Source: CAD feature listing. Evaluate the final solid. Frame: model axes, mm. A direction names the side the tool comes from. Give positions to 0.01 mm unless a question says otherwise; leave off trailing zeros. Write each loop counter-clockwise with the first axis right and the second up, starting at its lowest first coordinate (ties: lowest second). Pieces come first, ordered by that corner, then holes. Notation, with made-up numbers: (70.25, 42) -> (81.25, 42) arc R16 cw to (81.25, 56) -> close; hole circle Ø6 at (55, 82). An arc over 180 degrees is marked (long way). Use a Markdown table: item, result. Add a question column.
```python
from build123d import *

# Parameters (mm, degrees)
BOSS_EXTRUDE1_DEPTH = 45
BOSS_EXTRUDE2_START = -40
SKETCH1_3_R         = 10
BOSS_EXTRUDE2_DEPTH = 86
SKETCH1_4_R         = 10
BOSS_EXTRUDE3_DEPTH = 40
SKETCH1_5_R         = 25
BOSS_EXTRUDE4_DEPTH = 20
SKETCH2_R           = 5
BOSS_EXTRUDE5_DEPTH = 60
BOSS_EXTRUDE6_DEPTH = 10
SKETCH4_R           = 8
CUT_EXTRUDE2_DEPTH  = 15


with BuildPart() as part:
    # Sketch1 → Boss-Extrude1 (new body)
    with BuildSketch(Plane.XY):
        Polygon((15.533008589, 37.5), (-15.533008589, 37.5), (-37.5, 15.533008589), (-37.5, -15.533008589), (-15.533008589, -37.5), (15.533008589, -37.5), (37.5, -15.533008589), (37.5, 15.533008589), align=None)
    extrude(amount=BOSS_EXTRUDE1_DEPTH)

    # Sketch1<3> → Boss-Extrude2 (add)
    with BuildSketch(Plane.XY.offset(BOSS_EXTRUDE2_START)):
        with Locations((-15, 0)):
            Circle(SKETCH1_3_R)
    boss_extrude2 = extrude(amount=BOSS_EXTRUDE2_DEPTH)

    # Sketch1<4> → Boss-Extrude3 (add)
    with BuildSketch(Plane.XY):
        with Locations((15, 0)):
            Circle(SKETCH1_4_R)
    extrude(amount=-BOSS_EXTRUDE3_DEPTH)

    # Sketch1<5> → Boss-Extrude4 (add)
    with BuildSketch(Plane.XY):
        Circle(SKETCH1_5_R)
    extrude(amount=-BOSS_EXTRUDE4_DEPTH)

    # Sketch2 → Boss-Extrude5 (add)
    with BuildSketch(Plane(origin=(0, 0, -40), x_dir=(-1, 0, 0), z_dir=(0, 0, -1))):
        with Locations((15, 0)):
            Circle(SKETCH2_R)
    boss_extrude5 = extrude(amount=BOSS_EXTRUDE5_DEPTH)

    # Mirror2: Boss-Extrude5 across plane
    add(boss_extrude5.mirror(Plane(origin=(0, 0, 0), x_dir=(0, 0, 1), z_dir=(1, 0, 0))))

    # Sketch3 → Boss-Extrude6 (add)
    with BuildSketch(Plane(origin=(0, 0, -100), x_dir=(-1, 0, 0), z_dir=(0, 0, -1))):
        Polygon((-6.882058498, 0), (-9.259748515, 5.740251485), (-15, 8.117941502), (-20.740251485, 5.740251485), (-23.117941502, 0), (-20.740251485, -5.740251485), (-15, -8.117941502), (-9.259748515, -5.740251485), align=None)
    boss_extrude6 = extrude(amount=BOSS_EXTRUDE6_DEPTH)

    # Mirror3: Boss-Extrude6 across plane
    add(boss_extrude6.mirror(Plane(origin=(0, 0, 0), x_dir=(0, 0, 1), z_dir=(1, 0, 0))))

    # Mirror4: Boss-Extrude2 across plane
    add(boss_extrude2.mirror(Plane(origin=(0, 0, 0), x_dir=(0, 0, 1), z_dir=(1, 0, 0))))

    # Sketch4 → Cut-Extrude2 (cut)
    with BuildSketch(Plane.XY.offset(46)):
        with Locations((-15, 0)):
            Circle(SKETCH4_R)
    cut_extrude2 = extrude(amount=-CUT_EXTRUDE2_DEPTH, mode=Mode.SUBTRACT)

    # Mirror5: Cut-Extrude2 across plane
    add(cut_extrude2.mirror(Plane(origin=(0, 0, 0), x_dir=(0, 0, 1), z_dir=(1, 0, 0))), mode=Mode.SUBTRACT)


solid = part.part
```
(1) Cut plane A-A on x = 0. Return the cut outline in (y, z), then the cut area to 4 significant figures.
(2) Cut plane B-B on z = 24. Return the cut outline in (x, y), then the cut area to 3 significant figures.
(3) First-contact query: pin 1 Ø8 at (x, z) = (-22, 16) entering from +Y; pin 2 Ø10 at (y, z) = (-3, -75) entering from -X; pin 3 Ø12 at (y, z) = (14, -53) entering from +X; pin 4 Ø6 at (y, z) = (-24, -20.5) entering from -X. Flat tips, straight axial feed; report the tip coordinate or a pass-through.
(4) Cut plane C-C on z = -74. Return the cut outline in (x, y), then the cut area to 3 significant figures.
(5) Cut plane D-D on x = -17.5. Return the cut outline in (y, z), then the cut area to 3 significant figures.
(6) Access query for faces 1 (the flat face through (8.088, -2.91, -104.93)), 2 (the flat face through (-21.912, 2.91, -104.93)), 3 (the flat face through (17.83, 6.946, -104.93)), 4 (the cylindrical face through (-19.77, 1.5, -69.58)), 5 (the flat face through (-8.054, 2.83, -104.93)). Directions: +Z, -Z, +X, -X, +Y, -Y. A direction counts if a zero-diameter tool reaches every point of the face in a straight line with its end or side. Return the directions, or none.
(7) Mould query, pull axis Z, two halves, no side actions, for faces 6 (the flat face through (15, 0, 31)), 7 (the cylindrical face through (-5.46, 3, -30.14)), 8 (the flat face through (-13, 5, -40)). Classes: +Z half, -Z half, draft (parallel to the pull), parting line (faces both ways), or undercut.
(8) Material intervals for L1, parallel to Y at x = 15, z = 38.75; L2, parallel to Z at x = 17.5, y = -6.5; L3, parallel to Z at x = 1, y = 29, sorted ascending.
Output:
| question | item | result |
|---|---|---|
| 1 | outline | (-37.5, 0) -> (-25, 0) -> (-25, -20) -> (25, -20) -> (25, 0) -> (37.5, 0) -> (37.5, 45) -> (-37.5, 45) -> close |
| 1 | area | 4,375 mm^2 |
| 2 | outline | (-37.5, -15.53) -> (-15.53, -37.5) -> (15.53, -37.5) -> (37.5, -15.53) -> (37.5, 15.53) -> (15.53, 37.5) -> (-15.53, 37.5) -> (-37.5, 15.53) -> close |
| 2 | area | 4,660 mm^2 |
| 3 | pin 1 | y = 35.03 |
| 3 | pin 2 | x = -20 |
| 3 | pin 3 | through |
| 3 | pin 4 | x = -13.5 |
| 4 | outline | circle Ø10 at (-15, 0); circle Ø10 at (15, 0) |
| 4 | area | 157 mm^2 |
| 5 | outline | (-35.53, 0) -> (-17.85, 0) -> (-17.85, -20) -> (-9.68, -20) -> (-9.68, -40) -> (-4.33, -40) -> (-4.33, -100) -> (-7.08, -100) -> (-7.08, -110) -> (7.08, -110) -> (7.08, -100) -> (4.33, -100) -> (4.33, -40) -> (9.68, -40) -> (9.68, -20) -> (17.85, -20) -> (17.85, 0) -> (35.53, 0) -> (35.53, 45) -> (9.68, 45) -> (9.68, 46) -> (7.6, 46) -> (7.6, 31) -> (-7.6, 31) -> (-7.6, 46) -> (-9.68, 46) -> (-9.68, 45) -> (-35.53, 45) -> close |
| 5 | area | 4,750 mm^2 |
| 6 | face 1 | -Z, -Y |
| 6 | face 2 | -Z, -X, +Y |
| 6 | face 3 | -Z, +X, +Y |
| 6 | face 4 | none |
| 6 | face 5 | -Z, +Y |
| 7 | face 6 | +Z half |
| 7 | face 7 | draft |
| 7 | face 8 | undercut |
| 8 | L1 | -37.5 to -8, 8 to 37.5 |
| 8 | L2 | -110 to -100, -40 to 31 |
| 8 | L3 | 0 to 45 |
